Read the model definition and answer for the solid it produces. Units are mm, in the model's axes. Coordinates: 2 decimals unless noted, no trailing zeros. Loops run counter-clockwise (first coordinate to the right, second up) from the corner with the lowest first, then second, coordinate; pieces in that order, holes last.
from build123d import *

# Parameters (mm, degrees)
BOX224_W                  = 0.5
BOX224_H                  = 1
BOX224_DEPTH              = 11
BOX225_W                  = 0.5
BOX225_H                  = 1
BOX225_DEPTH              = 16
BOX225_ROLL_ANGLE         = 49
BOX226_W                  = 0.5
BOX226_H                  = 1
BOX226_DEPTH              = 16
BOX226_ROLL_ANGLE         = -49
BOX223_W                  = 0.5
BOX223_H                  = 1
BOX223_DEPTH              = 11
FUSION018_PLACEMENT_ANGLE = -32


with BuildPart() as cubo224:
    # Box224 → Box224 (new body)
    with BuildSketch(Plane(origin=(0, 12, 0.5), x_dir=(1, 0, 0), z_dir=(0, 0, 1))):
        with Locations((0.25, 0.5)):
            Rectangle(BOX224_W, BOX224_H)
    extrude(amount=BOX224_DEPTH)


with BuildPart() as cubo225:
    # Box225 → Box225 (new body)
    with BuildSketch(Plane.XY):
        with Locations((0.25, 0.5)):
            Rectangle(BOX225_W, BOX225_H)
    extrude(amount=BOX225_DEPTH)


with BuildPart() as cubo225_1:
    # Box225 roll: moved
    add(cubo225.part.rotate(Axis((0, 0, 0), (1, 0, 0)), BOX225_ROLL_ANGLE))


with BuildPart() as cubo225_2:
    # Box225 placement: moved
    add(cubo225_1.part.moved(Location((0, 12, 0.5))))


with BuildPart() as cubo226:
    # Box226 → Box226 (new body)
    with BuildSketch(Plane.XY):
        with Locations((0.25, 0.5)):
            Rectangle(BOX226_W, BOX226_H)
    extrude(amount=BOX226_DEPTH)


with BuildPart() as cubo226_1:
    # Box226 roll: moved
    add(cubo226.part.rotate(Axis((0, 0, 0), (1, 0, 0)), BOX226_ROLL_ANGLE))


with BuildPart() as cubo226_2:
    # Box226 placement: moved
    add(cubo226_1.part.moved(Location((0, 0.4, 1.3))))


with BuildPart() as fusion018:
    # Box223 → Box223 (new body)
    with BuildSketch(Plane.XY.offset(0.5)):
        with Locations((0.25, 0.5)):
            Rectangle(BOX223_W, BOX223_H)
    extrude(amount=BOX223_DEPTH)

    # Fusion018: union Cubo224, Cubo225, Cubo226
    add(cubo224.part)
    add(cubo225_2.part)
    add(cubo226_2.part)


with BuildPart() as fusion018_1:
    # Fusion018 placement: moved
    add(fusion018.part.moved(Location((-205, 113.4, 0))).rotate(Axis((-205, 113.4, 0), (0, 0, 1)), FUSION018_PLACEMENT_ANGLE))


solid = fusion018_1.part
Item 1: Determine the mould class of faces 1 (the face through (-202.783, 116.483, 8.962)), 2 (the face through (-199.868, 121.147, 2.856)), 3 (the face through (-199.704, 121.41, 7.971)) for opening direction Z: released by +Z, released by -Z, zero draft, split by the parting line, or undercut.
Numbers:
face 1: released by +Z
face 2: released by -Z
face 3: undercut
Item 2: A cutting plane is placed at C-C on z = 1.25. Determine the outline of the cut face in (x, y), then the cut area to 3 significant figures.
Numbers:
outline: (-205, 113.4) - (-204.58, 113.14) - (-203.59, 114.72) - (-204.01, 114.98) - close; (-199.1, 122.84) - (-198.67, 122.58) - (-197.69, 124.16) - (-198.11, 124.42) - close
area: 1.86 mm2
Item 3: A cutting plane is placed at D-D on x = -201.75. Determine the outline of the cut face in (y, z).
Numbers:
outline: (117.66, 4.26) - (118.6, 4.96) - (118.6, 6.93) - (117.66, 7.62) - (117.66, 6.3) - (118.14, 5.94) - (117.66, 5.59) - close
Item 4: A cutting plane is placed at A-A on z = 4.25. Determine the outline of the cut face in (x, y), then the cut area to 3 significant figures.
Numbers:
outline: (-205, 113.4) - (-204.58, 113.14) - (-204.05, 113.98) - (-204.47, 114.25) - close; (-202.99, 116.62) - (-202.57, 116.35) - (-201.76, 117.64) - (-202.18, 117.91) - close; (-200.93, 119.92) - (-200.5, 119.65) - (-199.7, 120.95) - (-200.12, 121.21) - close; (-198.64, 123.58) - (-198.22, 123.31) - (-197.69, 124.16) - (-198.11, 124.42) - close
area: 2.52 mm2
Item 5: Find the intervals of material crossed by line 1 along X through (y, z) = (123.75, 4.25); line 2 along Y through (x, z) = (-203.75, 1.75); line 3 along Y through (x, z) = (-202.5, 4), in increasing order.
Numbers:
line 1: x = -198.53 to -197.94
line 2: y = 114.46 to 115.4
line 3: y = 116.46 to 117.4
Item 6: Given pin 1 (4 mm diameter, centred on x = -200, z = 4, fed in from +Y); pin 2 (1.5 mm diameter, centred on x = -203.5, z = 4.5, fed in from -Y); pin 3 (2 mm diameter, centred on x = -203, z = 2, fed in from -Y), each flat-ended and moving along its own axis, determine where each tip first touches the part or whether it passes through.
Numbers:
pin 1: stops at y = 124.42
pin 2: stops at y = 113.66
pin 3: stops at y = 114.06
Item 7: A cutting plane is placed at B-B on y = 117. Determine the outline of the cut face in (x, z).
Numbers:
outline: (-202.75, 3.32) - (-202.16, 3.59) - (-202.16, 4.91) - (-202.75, 4.64) - close; (-202.75, 7.24) - (-202.16, 6.97) - (-202.16, 8.29) - (-202.75, 8.57) - close
